Here's how the part is built. I have some questions about the finished solid (model axes, mm). A direction names the side the tool comes from. Round coordinates to 2 decimals unless told otherwise and drop trailing zeros. Order: outer loops, then holes, each group sorted by start corner. A loop starts at its lowest first (then second) coordinate and runs counter-clockwise, first axis right, second up. Notation, with made-up numbers: (-10.75, 45) - (36.25, 45) arc R4 ccw to (36.25, 52) - close; hole circle Ø10 at (46, 15.5). An arc over 180 degrees is marked (long way). One line per item, written item: value.
Autodesk Inventor part; units mm, degrees
ref_plane "YZ Plane" through (0, 0, 0) normal (1, 0, 0) x (0, 1, 0)
ref_plane "XZ Plane" through (0, 0, 0) normal (0, 1, 0) x (-1, 0, 0)
ref_plane "XY Plane" through (0, 0, 0) normal (0, 0, 1) x (1, 0, 0)
sketch "Sketch1" plane through (0, 0, 0) normal (0, 1, 0) x (-1, 0, 0)
  line L0 (0, 0) -> (60, 0) construction
  line L1 (60, 0) -> (60, -25) construction
  line L2 (60, -25) -> (0, -25) construction
  line L3 (0, -25) -> (0, 0) construction
  line L4 (60.5, 0.5) -> (-0.5, 0.5)
  line L5 (-0.5, 0.5) -> (-0.5, -25.5)
  line L6 (-0.5, -25.5) -> (60.5, -25.5)
  line L7 (60.5, -25.5) -> (60.5, 0.5)
  circle A0 centre (53, -19) radius 2.5
  circle A1 centre (7, -19) radius 2.5
  circle A2 centre (7, -6) radius 2.5
  circle A3 centre (53, -6) radius 2.5
  line L8 (53, -19) -> (7, -19) construction
  line L9 (7, -19) -> (7, -6) construction
  line L10 (60.5, 0.5) -> (60.5, 20.5)
  line L11 (60.5, 20.5) -> (-0.5, 20.5)
  line L12 (-0.5, 20.5) -> (-0.5, 0)
  line L13 (89.6876, -43.5705) -> (-21.1545, -43.5705)
  line L14 (-21.1545, -43.5705) -> (-21.1545, 42.1657)
  line L15 (-21.1545, 42.1657) -> (89.6876, 42.1657)
  line L16 (89.6876, 42.1657) -> (89.6876, -43.5705)
  point P0 (30, -19)
  point P1 (30, -25)
  point P2 (7, -12.5)
  point P3 (0, -12.5)
  point P4 (-0.5, 0.5)
  point P5 (-0.5, 0.5)
  dimension "d0" = 25
  dimension "d1" = 60
  dimension "d2" = 0.5
  dimension "d3" = 0.5
  dimension "d4" = 0.5
  dimension "d5" = 0.5
  dimension "d6" = 5
  dimension "d7" = 46
  dimension "d8" = 13
  dimension "d72" = 20
sketch "Sketch2" plane through (0, 0, 0) normal (0, 1, 0) x (-1, 0, 0)
  line L0 (-5.4, 29) -> (65.4, 29)
  line L1 (65.4, 29) -> (65.4, -26)
  line L2 (65.4, -26) -> (-5.4, -26)
  line L3 (-5.4, -26) -> (-5.4, 29)
  line L4 (60.5, -25.5) -> (60.5, 0.5) construction
  line L5 (-0.5, 0.5) -> (-0.5, -25.5) construction
  line L6 (-0.5, -25.5) -> (60.5, -25.5) construction
  point P0 (0, 0)
  point P1 (60.5, -12.5)
  point P2 (65.4, 1.5)
  point P3 (30, -26)
  point P4 (30, -25.5)
  point P5 (30, -53.5)
  point P6 (110, 1.5)
  dimension "d9" = 70.8
  dimension "d10" = 55
  dimension "d50" = 35.4
  dimension "d74" = 13.5
extrude "Extrusion1" add sketch "Sketch2" against normal blind 35.4
extrude "Extrusion2" cut sketch "Sketch1" along normal blind 10 and the other way blind 5 contours L7 L6 L5 L4 | L4 L12 L11 L10 | L13 L14 L15 L16
extrude "Extrusion3" cut sketch "Sketch1" along normal blind 10 and the other way blind 30.4 contours A0 | A1 | A2 | A3
sketch "Sketch3" plane through (5.4, -35.4, -26) normal (0, 0, -1) x (1, 0, 0)
  line L0 (-70.8, 0) -> (-70.8, 17.5)
  line L1 (-70.8, 17.5) -> (-61.3, 17.5)
  line L2 (-61.3, 17.5) -> (-61.3, 3.175)
  line L3 (0, 0) -> (0, 17.5)
  line L4 (0, 17.5) -> (-9.5, 17.5)
  line L5 (-9.5, 17.5) -> (-9.5, 3.175)
  arc A0 (-61.3, 3.175) -> (-58.125, 0) centre (-58.125, 3.175) ccw
  arc A1 (-12.675, 0) -> (-9.5, 3.175) centre (-12.675, 3.175) ccw
  line L6 (0, 0) -> (-12.675, 0)
  line L7 (-70.8, -35.4) -> (-70.8, 0)
  line L8 (-70.8, 0) -> (0, 0)
  line L9 (-58.125, 0) -> (-70.8, 0)
  point P0 (-61.3, 0)
  dimension "d67" = 3.175
  dimension "d68" = 9.5
  dimension "d69" = 17.5
  dimension "d70" = 90
  dimension "d71" = 90
extrude "Extrusion4" add sketch "Sketch3" against normal up to surface (55 mm away)
sketch "Sketch4" plane through (0, -5, 0) normal (0, 1, 0) x (1, 0, 0)
  circle A0 centre (-45.5, -17.5) radius 3.413
  circle A1 centre (-14.5, -17.5) radius 3.413
  line L0 (-45.5, -17.5) -> (-14.5, -17.5) construction
  line L1 (-65.4, 26) -> (5.4, 26)
  line L2 (-45.5, -17.5) -> (-45.5, 12.5) construction
  line L3 (-45.5, 12.5) -> (-14.5, 12.5) construction
  line L4 (-14.5, 12.5) -> (-14.5, -17.5) construction
  circle A2 centre (-45.5, 12.5) radius 3.413
  circle A3 centre (-14.5, 12.5) radius 3.413
  point P0 (-30, -17.5)
  point P1 (-30, 26)
  dimension "d29" = 6.826
  dimension "d78" = 30
  dimension "d79" = 31
  dimension "d80" = 13.5
extrude "Extrusion5" cut sketch "Sketch4" against normal blind 36.5125
sketch "Sketch5" plane through (0, -5, 0) normal (0, 1, 0) x (1, 0, 0)
  circle A0 centre (-45.5, -17.5) radius 3.413 construction
  circle A1 centre (-14.5, -17.5) radius 3.413 construction
  circle A2 centre (-14.5, -17.5) radius 6
  circle A3 centre (-45.5, -17.5) radius 6
  circle A4 centre (-45.5, 12.5) radius 6
  circle A5 centre (-14.5, 12.5) radius 6
  circle A6 centre (-14.5, 12.5) radius 3.413
  circle A7 centre (-45.5, 12.5) radius 3.413
  point P0 (0, 0)
  point P1 (-43.1765, -26)
  point P2 (-47.8235, -26)
  point P3 (-12.1765, -26)
  point P4 (-16.8235, -26)
  dimension "d34" = 12
extrude "Extrusion6" cut sketch "Sketch5" against normal blind 6 contours A2 | A3 | A4 | A5 | A6
sketch "Sketch8" plane through (-52.725, -35.4, 29) normal (0, 0, 1) x (-1, 0, 0)
  line L0 (-22.725, 0) -> (-13.725, 0)
  line L1 (-13.725, 0) -> (-12.725, 1)
  line L2 (-12.725, 1) -> (-12.725, 4)
  line L3 (-12.725, 4) -> (-16.175, 7.45)
  line L4 (-16.175, 7.45) -> (-16.175, 9.8767)
  line L5 (-16.175, 9.8767) -> (-14.9578, 11.0939)
  arc A0 (-13.2458, 12.8058) -> (-14.9578, 11.0939) centre (-12.9761, 10.8241) ccw
  line L6 (-13.2458, 12.8058) -> (-12.725, 13.3267)
  line L7 (-12.725, 13.3267) -> (-12.725, 14.66)
  line L8 (-12.725, 14.66) -> (-13.2458, 15.1808)
  arc A1 (-14.9578, 16.8928) -> (-13.2458, 15.1808) centre (-12.9761, 17.1626) ccw
  line L9 (-14.9578, 16.8928) -> (-15.565, 17.5)
  line L10 (-15.565, 17.5) -> (-22.725, 17.5)
  line L11 (-22.725, 17.5) -> (-22.725, 0) construction
  line L12 (-14.9578, 11.0939) -> (-13.2458, 12.8058) construction
  line L13 (-14.9578, 16.8928) -> (-13.2458, 15.1808) construction
  line L14 (-29.275, 7.45) -> (-29.275, 9.8767)
  line L15 (-29.275, 9.8767) -> (-30.4922, 11.0939)
  line L16 (-30.4922, 11.0939) -> (-32.2042, 12.8058) construction
  arc A2 (-30.4922, 11.0939) -> (-32.2042, 12.8058) centre (-32.4739, 10.8241) ccw
  line L17 (-32.2042, 12.8058) -> (-32.725, 13.3267)
  line L18 (-32.725, 13.3267) -> (-32.725, 14.66)
  line L19 (-32.725, 14.66) -> (-32.2042, 15.1808)
  line L20 (-30.4922, 16.8928) -> (-32.2042, 15.1808) construction
  arc A3 (-32.2042, 15.1808) -> (-30.4922, 16.8928) centre (-32.4739, 17.1626) ccw
  line L21 (-29.885, 17.5) -> (-22.725, 17.5)
  line L22 (-30.4922, 16.8928) -> (-29.885, 17.5)
  line L23 (-32.725, 4) -> (-29.275, 7.45)
  line L24 (-22.725, 0) -> (-31.725, 0)
  line L25 (-32.725, 1) -> (-32.725, 4)
  line L26 (-31.725, 0) -> (-32.725, 1)
  line L27 (-13.725, 0) -> (-12.725, 0)
  line L28 (-12.725, 1) -> (-12.725, 0)
  line L29 (-32.725, 1) -> (-32.725, 0)
  line L30 (-32.725, 0) -> (-31.725, 0)
  line L31 (-13.725, 0) -> (-12.725, -1)
  line L32 (-12.725, -1) -> (-12.725, -4)
  line L33 (-16.175, -7.45) -> (-16.175, -9.8767)
  line L34 (-12.725, -4) -> (-16.175, -7.45)
  line L35 (-12.725, -1) -> (-12.725, 0)
  line L36 (-31.725, 0) -> (-32.725, -1)
  line L37 (-32.725, -4) -> (-29.275, -7.45)
  line L38 (-32.2042, -12.8058) -> (-32.725, -13.3267)
  line L39 (-32.725, -13.3267) -> (-32.725, -14.66)
  line L40 (-29.275, -7.45) -> (-29.275, -9.8767)
  line L41 (-32.725, -14.66) -> (-32.2042, -15.1808)
  line L42 (-30.4922, -11.0939) -> (-32.2042, -12.8058) construction
  arc A4 (-32.2042, -12.8058) -> (-30.4922, -11.0939) centre (-32.4739, -10.8241) ccw
  line L43 (-29.275, -9.8767) -> (-30.4922, -11.0939)
  line L44 (-30.4922, -16.8928) -> (-32.2042, -15.1808) construction
  arc A5 (-30.4922, -16.8928) -> (-32.2042, -15.1808) centre (-32.4739, -17.1626) ccw
  line L45 (-30.4922, -16.8928) -> (-29.885, -17.5)
  line L46 (-29.885, -17.5) -> (-22.725, -17.5)
  line L47 (-22.725, -17.5) -> (-22.725, 0) construction
  line L48 (-32.725, -1) -> (-32.725, 0)
  line L49 (-32.725, -1) -> (-32.725, -4)
  line L50 (-16.175, -9.8767) -> (-14.9578, -11.0939)
  line L51 (-14.9578, -11.0939) -> (-13.2458, -12.8058) construction
  arc A6 (-14.9578, -11.0939) -> (-13.2458, -12.8058) centre (-12.9761, -10.8241) ccw
  line L52 (-13.2458, -12.8058) -> (-12.725, -13.3267)
  line L53 (-12.725, -13.3267) -> (-12.725, -14.66)
  line L54 (-12.725, -14.66) -> (-13.2458, -15.1808)
  line L55 (-15.565, -17.5) -> (-22.725, -17.5)
  line L56 (-14.9578, -16.8928) -> (-13.2458, -15.1808) construction
  arc A7 (-13.2458, -15.1808) -> (-14.9578, -16.8928) centre (-12.9761, -17.1626) ccw
  line L57 (-14.9578, -16.8928) -> (-15.565, -17.5)
  line L58 (-45.45, 0) -> (0, 0)
  point P0 (-52.725, -35.4)
  point P1 (-12.725, 2.5)
  point P2 (-32.725, 0.5)
  point P3 (-12.725, -2.5)
  point P4 (-32.725, -0.5)
  dimension "d51" = 1
  dimension "d52" = 3
  dimension "d53" = 135
  dimension "d54" = 2
  dimension "d55" = 3.45
  dimension "d56" = 17.5
  dimension "d57" = 7.16
  dimension "d58" = 2.375
  dimension "d59" = 1.3333
  dimension "d60" = 2.4211
  dimension "d61" = 10
extrude "Extrusion9" cut sketch "Sketch8" against normal up to surface (55 mm away) contours L0 L31 L32 L34 L33 L50 A6 L52 L53 L54 A7 L57 L55 L46 L45 A5 L41 L39 L38 A4 L43 L40 L37 L49 L36 L24 | L27 L35 L31 | L36 L48 L30
sketch "Sketch10" plane through (-65.4, -5, 29) normal (0, 0, 1) x (1, 0, 0)
  arc A0 (12.675, -30.4) -> (9.5, -33.575) centre (12.675, -33.575) ccw
  line L0 (0, 0) -> (0, -47.9)
  line L1 (70.8, 0) -> (0, 0)
  line L2 (9.5, -33.575) -> (9.5, -30.4)
  line L3 (9.5, -30.4) -> (12.675, -30.4)
  line L4 (9.5, -47.9) -> (0, -47.9)
  line L5 (0, -47.9) -> (9.5, -47.9)
  line L6 (9.5, -47.9) -> (9.5, -33.575)
  line L7 (44.9, -6) -> (56.9, -6)
  line L8 (45.4, -26.4) -> (45.4, -30.4)
  line L9 (58.125, -30.4) -> (45.4, -30.4)
  arc A1 (61.3, -33.575) -> (58.125, -30.4) centre (58.125, -33.575) ccw
  line L10 (61.3, -47.9) -> (61.3, -33.575)
  line L11 (70.8, -47.9) -> (61.3, -47.9)
  line L12 (70.8, 0) -> (70.8, -47.9)
  line L13 (70.8, 0) -> (0, 0)
  line L14 (0, 0) -> (0, -47.9)
  line L15 (9.5, -47.9) -> (0, -47.9)
  line L16 (9.5, -33.575) -> (9.5, -47.9)
  arc A2 (12.675, -30.4) -> (9.5, -33.575) centre (12.675, -33.575) ccw
  line L17 (25.4, -30.4) -> (12.675, -30.4)
  line L18 (25.4, -30.4) -> (25.4, -26.4)
  line L19 (25.4, -26.4) -> (28.85, -22.95)
  line L20 (28.85, -22.95) -> (28.85, -20.5233)
  line L21 (28.85, -20.5233) -> (27.6328, -19.3061)
  arc A3 (27.6328, -19.3061) -> (25.9208, -17.5942) centre (25.6511, -19.5759) ccw
  line L22 (25.9208, -17.5942) -> (25.4, -17.0733)
  line L23 (25.4, -17.0733) -> (25.4, -15.74)
  line L24 (25.4, -15.74) -> (25.9208, -15.2192)
  arc A4 (25.9208, -15.2192) -> (27.6328, -13.5072) centre (25.6511, -13.2374) ccw
  line L25 (27.6328, -13.5072) -> (28.24, -12.9)
  line L26 (28.24, -12.9) -> (42.56, -12.9)
  line L27 (42.56, -12.9) -> (43.1672, -13.5072)
  arc A5 (43.1672, -13.5072) -> (44.8792, -15.2192) centre (45.1489, -13.2374) ccw
  line L28 (44.8792, -15.2192) -> (45.4, -15.74)
  line L29 (45.4, -15.74) -> (45.4, -17.0733)
  line L30 (45.4, -17.0733) -> (44.8792, -17.5942)
  arc A6 (44.8792, -17.5942) -> (43.1672, -19.3061) centre (45.1489, -19.5759) ccw
  line L31 (43.1672, -19.3061) -> (41.95, -20.5233)
  line L32 (41.95, -20.5233) -> (41.95, -22.95)
  line L33 (41.95, -22.95) -> (45.4, -26.4)
  line L34 (58.125, -30.4) -> (61.3, -30.4)
  line L35 (61.3, -30.4) -> (61.3, -33.575)
  line L36 (9.5, -30.4) -> (6.4, 0)
  line L37 (0, 0) -> (70.8, 0)
  line L38 (61.3, -30.4) -> (64.4, 0)
  line L39 (6.4, 0) -> (6.4, -12)
  line L40 (6.4, -12) -> (9.5, -30.4)
  line L41 (61.3, -30.4) -> (64.4, -12)
  line L42 (64.4, -12) -> (64.4, 0)
  point P0 (65.4, 5)
  point P1 (64.4, 0)
  point P2 (6.4, 0)
  point P3 (6.4, 0)
  point P4 (64.4, 0)
  dimension "d86" = 58
  dimension "d101" = 12
extrude "Extrusion10" cut sketch "Sketch10" against normal through all contours A0 L2 L3 | L6 L4 L0 L1 L39 L40 L2 | L1 L12 L11 L10 L35 L41 L42 | L35 A1 L34
sketch "Sketch11" plane through (-37.16, -17.9, 29) normal (0, 0, 1) x (1, 0, 0)
  line L0 (-18.74, -17.5) -> (-2.84, -17.5)
  line L1 (-3.04, -17.5) -> (17.36, -17.5)
  line L2 (17.36, -17.5) -> (17.36, 0.1)
  line L3 (17.36, 0.1) -> (-3.04, 0.1)
  line L4 (-3.04, 0.1) -> (-3.04, -17.5)
  line L5 (-2.84, -17.5) -> (-2.84, -13.5)
  line L6 (17.16, -13.5) -> (17.16, -17.5)
  line L7 (0, 0) -> (14.32, 0)
  point P0 (37.16, 17.9)
  point P1 (-16.7296, -17.5)
  point P2 (-2.84, -15.5)
  dimension "d88" = 0.2
  dimension "d89" = 0.2
  dimension "d90" = 0.1
extrude "Extrusion11" add sketch "Sketch11" against normal up to surface (55 mm away)
sketch "Sketch12" plane through (0, 0, 0) normal (1, 0, 0) x (0, 1, 0)
  line L0 (-5, 5.8394) -> (-10, 29)
  line L1 (-35.4, 29) -> (-5, 29)
  line L2 (-5, 29) -> (-5, -26)
  point P0 (0, 0)
  dimension "d93" = 5
extrude "Extrusion12" cut sketch "Sketch12" against normal through all
sketch "Sketch13" plane through (-14.5, -11, 17.5) normal (0, 1, 0) x (1, 0, 0)
  circle A0 centre (0, 0) radius 3.413
  circle A1 centre (0, 0) radius 6
  circle A2 centre (-31, 0) radius 3.413
  circle A3 centre (-31, 0) radius 3.413
  circle A4 centre (-31, 0) radius 6
  point P0 (14.5, 17.5)
extrude "Extrusion13" cut sketch "Sketch13" against normal blind 5
chamfer "Chamfer2" distance 1 angle 45 6 edges at (-30, -10, 29) (-30, -5, -26) (-1, -7.5, 17.4197) (-59, -7.5, 17.4197) (-59, -5, -10.0803) (-1, -5, -10.0803)
properties part number "BK12_Spacer_Metal"
Q1. If I drill on line 1 along Z through (x, y) = (-45.5, -19.5); line 2 along Z through (x, y) = (-53, -25); line 3 along X through (y, z) = (-12, -7), over which ranges is the centre line in solid material (lowest first)?
Results list:
line 1: -26 to -15.91, -9.09 to 14.09, 20.91 to 29
line 2: -26 to -21.5, -16.5 to -8.5, -3.5 to 29
line 3: -59 to -55.29, -50.71 to -9.29, -4.71 to -1
Q2. If we section it at A-A, the plane y = -13: Give the number of separate pieces and of enclosed holes in the cut face, then the cut area to 3 significant figures.
Results list:
separate pieces: 1
enclosed holes: 8
area: 2,810 mm²
Q3. If we section it at C-C, the plane z = 17.5: Please give me the cut outline in (x, y), then the cut area to 3 significant figures.
Results list:
outline: (-59, -17) - (-55.9, -35.4) - (-48.91, -35.4) - (-48.91, -16) - (-51.5, -16) - (-51.5, -7.52) - (-58, -7.52) - (-59, -8.54) - close; (-42.09, -35.4) - (-17.91, -35.4) - (-17.91, -16) - (-20.5, -16) - (-20.5, -7.52) - (-39.5, -7.52) - (-39.5, -16) - (-42.09, -16) - close; (-11.09, -35.4) - (-4.1, -35.4) - (-1, -17) - (-1, -8.54) - (-2, -7.52) - (-8.5, -7.52) - (-8.5, -16) - (-11.09, -16) - close
area: 1,090 mm²
Q4. If we section it at D-D, the plane x = -7: Please give me the cut outline in (y, z), then the cut area to 3 significant figures.
Results list:
outline: (-35.4, -26) - (-6, -26) - (-5, -25) - (-5, -21.5) - (-30.4, -21.5) - (-30.4, -16.5) - (-5, -16.5) - (-5, -8.5) - (-30.4, -8.5) - (-30.4, -3.5) - (-5, -3.5) - (-5, 5.84) - (-9.79, 28.02) - (-11, 29) - (-35.4, 29) - close
area: 1,360 mm²
Q5. Will these pins go through, and if not, where does the flat tip stop? pin 1 (3.5 mm diameter, centred on x = -14, z = -12.5, fed in from +Y); pin 2 (9.5 mm diameter, centred on x = -44.5, z = 17.5, fed in from +Y); pin 3 (1.5 mm diameter, centred on x = -52, z = -19.5, fed in from +Y); pin 4 (8 mm diameter, centred on x = -14, z = 15, fed in from +Y).
Results list:
pin 1: through
pin 2: y = -16
pin 3: y = -30.4
pin 4: y = -6.11
Q6. If we section it at B-B, the plane x = -45.5: Please give me the cut outline in (y, z).
Results list:
outline: (-35.4, -26) - (-6, -26) - (-5, -25) - (-5, -18.5) - (-11, -18.5) - (-11, -15.91) - (-35.4, -15.91) - close; (-35.4, -9.09) - (-11, -9.09) - (-11, -6.5) - (-5, -6.5) - (-5, 5.84) - (-6.22, 11.5) - (-16, 11.5) - (-16, 14.09) - (-35.4, 14.09) - close; (-35.4, 20.91) - (-16, 20.91) - (-16, 23.5) - (-8.81, 23.5) - (-9.79, 28.02) - (-11, 29) - (-35.4, 29) - close
Q7. Which directions (+Z, -Z, +X, -X, +Y, -Y) give clear straight access to the entire face, cutting with the end or side of a thin tool? Please do faces 1 (the cylindrical face through (-8.96, -7.96, -10.2)), 2 (the flat face through (-2.57, -26.33, 1.89)).
Results list:
face 1: +Y
face 2: +Z, -Z, +X, -Y
